Check sheet for the modelled part. Datum: model origin and axes. Units: mm. A direction names the side the tool comes from. Coordinates: 2 decimals unless noted, no trailing zeros. Use CSV: the item, a comma, the result in double quotes. Start each with the question number.
(1) Set-up check for faces 1 (the flat face through (-75, 0, 44)), 2 (the flat face through (-1, 2, 5.228)): record each of +Z, -Z, +X, -X, +Y, -Y from which the full face is reachable in a straight line by a thin tool's end or side.
(2) Go/stop test with flat-tipped pins: pin 1 Ø1.8 at (x, y) = (21.5, 0.5) entering from -Z; pin 2 Ø5 at (x, z) = (-70.96, 85.95) entering from -Y; pin 3 Ø3 at (x, z) = (70.96, 3.53) entering from -Y; pin 4 Ø4.5 at (x, z) = (70.96, 85.95) entering from +Y. Record where each tip stops, or that it passes through.
(3) Scan lines: line 1 (X direction, y = 1.5, z = 11.5); line 2 (Z direction, x = -4, y = 1). Record each from-to range of solid material in increasing order.
(4) Draft check along Z on faces 3 (the flat face through (1, 3, 0)), 4 (the flat face through (67.487, -1, 44)), 5 (the cylindrical face through (-69.054, 1.999, 4.127)), 6 (the flat face through (75, 0, 46)). Enter one of: pulls with the +Z half, pulls with the -Z half, needs draft (parallel to the pull), parting line crosses it, or undercut.
from build123d import *

# Parameters (mm, degrees)
F1_DEPTH = 75
F2_DEPTH = 75
F4_W     = 135
F4_H     = 78
F5_DEPTH = 12
F6_R     = 2
F7_DEPTH = 25


with BuildPart() as f1:
    # F0 (on Right) → F1 (new body)
    with BuildSketch(Plane.YZ):
        with BuildLine():
            Line((6, 90), (0, 90))
            add(Edge.make_bspline(
                [(0, 90), (-5.988211, 73.405368), (-6, 18), (0, 0)],
                knots=[0, 0, 0, 0, 90, 90, 90, 90], degree=3))
            Line((0, 0), (6, 0))
            add(Edge.make_bspline(
                [(6, 90), (0, 73.029437), (0, 18), (6, 0)],
                knots=[0, 0, 0, 0, 90, 90, 90, 90], degree=3))
        make_face()
    extrude(amount=F1_DEPTH)

    # F1_face (on face) → F2 (join)
    with BuildSketch(Plane(origin=(0, -0.249906, 45.026938), x_dir=(0, 1, 0), z_dir=(-1, 0, 0))):
        with BuildLine():
            Line((0.249906, -44.973062), (6.249906, -44.973062))
            add(Edge.make_bspline(
                [(6.249906, -44.973062), (0.249906, -28.002499), (0.249906, 27.026938), (6.249906, 45.026938)],
                knots=[0, 0, 0, 0, 90, 90, 90, 90], degree=3))
            Line((6.249906, 45.026938), (0.249906, 45.026938))
            add(Edge.make_bspline(
                [(0.249906, -44.973062), (-5.738305, -28.37843), (-5.750094, 27.026938), (0.249906, 45.026938)],
                knots=[0, 0, 0, 0, 90, 90, 90, 90], degree=3))
        make_face()
    extrude(amount=F2_DEPTH)

    # F4 (on offset) → F5 (cut)
    with BuildSketch(Plane.XZ.offset(6)):
        with Locations((-0.013318, 44.228188)):
            Rectangle(F4_W, F4_H)
    extrude(amount=-F5_DEPTH, mode=Mode.SUBTRACT)

    # F6 (on offset) → F7 (cut)
    with BuildSketch(Plane.XZ.offset(6)):
        with Locations((-70.961185, 85.947864)):
            Circle(F6_R)
        with Locations((70.961185, 85.947864)):
            Circle(F6_R)
        with Locations((70.961185, 3.526589)):
            Circle(F6_R)
        with Locations((-70.961185, 3.526589)):
            Circle(F6_R)
    extrude(amount=-F7_DEPTH, mode=Mode.SUBTRACT)


solid = f1.part
Outcome:
1,face 1,"+Z, -Z, -X, +Y, -Y"
1,face 2,"+Y, -Y"
2,pin 1,"stops at z = 0"
2,pin 2,"stops at y = -1.71"
2,pin 3,"passes through"
2,pin 4,"stops at y = 5.43"
3,line 1,"x = -75 to -67.51, 67.49 to 75"
3,line 2,"z = 0 to 5.23, 83.23 to 90"
4,face 3,"pulls with the -Z half"
4,face 4,"undercut"
4,face 5,"undercut"
4,face 6,"needs draft"
